from build123d import *

# Parameters (mm, degrees)
BOSS_EXTRUDE1_DEPTH = 1.6
SKETCH2_W           = 112.5
SKETCH2_H           = 91.209934792
BOSS_EXTRUDE2_DEPTH = 38
SKETCH3_W           = 129
SKETCH3_H           = 3
BOSS_EXTRUDE3_DEPTH = 38
SKETCH4_R           = 1.5
SKETCH4_R_2         = 1.75
CUT_EXTRUDE1_DEPTH  = 4
SKETCH5_R           = 1.75
SKETCH5_R_2         = 1.5
CUT_EXTRUDE2_DEPTH  = 4
FILLET1_R           = 2
FILLET2_R           = 2
FILLET3_R           = 2


with BuildPart() as part:
    # Sketch1 → Boss-Extrude1 (new body)
    with BuildSketch(Plane(origin=(0, 0, 0), x_dir=(1, 0, 0), z_dir=(0, 1, 0))):
        with BuildLine():
            Line((-68.019736842, 49), (-68.019736842, -49))
            Line((-68.019736842, -49), (60.980263158, -49))
            Line((60.980263158, -49), (60.980263158, -46))
            Line((60.980263158, -46), (54.480263158, -46))
            Line((54.480263158, -46), (54.480263158, 40.25))
            ThreePointArc((54.480263158, 40.25), (52.730263158, 42), (54.480263158, 43.75))
            Line((54.480263158, 43.75), (60.980263158, 43.75))
            Line((60.980263158, 43.75), (60.980263158, 49))
            Line((60.980263158, 49), (-68.019736842, 49))
        make_face()
    extrude(amount=BOSS_EXTRUDE1_DEPTH)

    # Sketch2 → Boss-Extrude2 (add)
    with BuildSketch(Plane(origin=(0, 1.6, 0), x_dir=(1, 0, 0), z_dir=(0, 1, 0))):
        with Locations((-5.269736842, -0.395032604)):
            Rectangle(SKETCH2_W, SKETCH2_H)
    extrude(amount=BOSS_EXTRUDE2_DEPTH)

    # Sketch3 → Boss-Extrude3 (add)
    with BuildSketch(Plane(origin=(0, 1.6, 0), x_dir=(1, 0, 0), z_dir=(0, 1, 0))):
        with Locations((-3.519736842, -47.5)):
            Rectangle(SKETCH3_W, SKETCH3_H)
    extrude(amount=BOSS_EXTRUDE3_DEPTH)

    # Sketch4 → Cut-Extrude1 (cut)
    with BuildSketch(Plane.XY.offset(49)):
        with Locations((-36.019736842, 21.1)):
            Circle(SKETCH4_R)
        with Locations((40.980263158, 12.1)):
            Circle(SKETCH4_R)
        with Locations((40.980263158, 30.1)):
            Circle(SKETCH4_R)
        with Locations((-61.519736842, 30.6)):
            Circle(SKETCH4_R_2)
    extrude(amount=-CUT_EXTRUDE1_DEPTH, mode=Mode.SUBTRACT)

    # Sketch5 → Cut-Extrude2 (cut)
    with BuildSketch(Plane.XZ):
        with Locations(Location((-63.519736842, 43.5, 0), (0, 0, 270))):
            Circle(SKETCH5_R)
        with Locations(Location((9.980263158, 18, 0), (0, 0, 270))):
            Circle(SKETCH5_R_2)
        with Locations(Location((9.980263158, -15, 0), (0, 0, 270))):
            Circle(SKETCH5_R_2)
    extrude(amount=-CUT_EXTRUDE2_DEPTH, mode=Mode.SUBTRACT)

    # Fillet1
    fillet1_edges = [part.edges().sort_by_distance(p)[0] for p in [
        (60.980263158, 0.8, -49),
    ]]
    fillet(fillet1_edges, radius=FILLET1_R)

    # Fillet2
    fillet2_edges = [part.edges().sort_by_distance(p)[0] for p in [
        (60.980263158, 39.6, 47.5),
    ]]
    fillet(fillet2_edges, radius=FILLET2_R)

    # Fillet3
    fillet3_edges = [part.edges().sort_by_distance(p)[0] for p in [
        (-68.019736842, 39.6, 47.5),
    ]]
    fillet(fillet3_edges, radius=FILLET3_R)


solid = part.part
Could you check a few things on this model? Use its own coordinates, in mm. A direction names the side the tool comes from. Give positions to 0.01 mm unless a question says otherwise; leave off trailing zeros. Order: outer loops, then holes, each group sorted by start corner. A loop starts at its lowest first (then second) coordinate and runs counter-clockwise, first axis right, second up.
1. Suppose I cut it at A-A (z = 43.5). List the corners of the cut face in (x, y) for me, plus the area to 3 significant figures.
2. I need wall thicknesses on L1, parallel to X at y = 2, z = -15; L2, parallel to Z at x = -52, y = 37; L3, parallel to X at y = 22, z = 21. Which ranges of each line are inside material? Lowest first, please.
3. Suppose I cut it at B-B (y = 21.1). List the corners of the cut face in (x, z) for me, plus the area to 3 significant figures.
4. Suppose I cut it at C-C (x = -18). List the corners of the cut face in (y, z) for me, plus the area to 3 significant figures.
5. Suppose I cut it at D-D (z = 18). List the corners of the cut face in (x, y) for me, plus the area to 3 significant figures.
6. We'd pull the mould along X, two halves only. Please class faces 1 (the cylindrical face through (10, 2, 19.5)), 2 (the flat face through (-68.02, 1, 22)), 3 (the flat face through (56, 20, 46)): pulls with the +X half, pulls with the -X half, needs draft (parallel to the pull), parting line crosses it, or undercut.
7. Will these pins go through, and if not, where does the flat tip stop? P1, Ø5, axis at x = -65, y = 30, coming from the -Z side; P2, Ø2.5, axis at x = 40.98, y = 30.1, coming from the +Z side; P3, Ø1, axis at x = -37.5, z = -15, coming from the -Y side; P4, Ø4, axis at y = 16.5, z = -33, coming from the -X side.
8. For faces 4 (the flat face through (41, 12, 45)), 5 (the flat face through (10, 4, -15)), 6 (the flat face through (-4, 1.6, -47)), 7 (the flat face through (-6, 20, -45.21)), which set-ups out of +Z, -Z, +X, -X, +Y, -Y let a thin tool reach every point of the face, with its end or its side?
Solved:
1. outline: (-68.02, 0) - (-65.27, 0) - (-65.27, 1.6) - (-68.02, 1.6) - close; (-61.77, 0) - (54.48, 0) - (54.48, 1.6) - (50.98, 1.6) - (50.98, 39.6) - (-61.52, 39.6) - (-61.52, 1.6) - (-61.77, 1.6) - close
1. area: 4,470 mm2
2. L1: x = -61.52 to 8.48, 11.48 to 50.98
2. L2: z = -45.21 to 49
2. L3: x = -61.52 to 50.98
3. outline: (-68.02, 46) - (-61.52, 46) - (-61.52, -45.21) - (50.98, -45.21) - (50.98, 46) - (60.98, 46) - (60.98, 49) - (-34.52, 49) - (-34.52, 45) - (-37.52, 45) - (-37.52, 49) - (-68.02, 49) - close
3. area: 10,600 mm2
4. outline: (0, -49) - (1.6, -49) - (1.6, -45.21) - (39.6, -45.21) - (39.6, 49) - (0, 49) - close
4. area: 3,740 mm2
5. outline: (-68.02, 0) - (8.48, 0) - (8.48, 4) - (11.48, 4) - (11.48, 0) - (54.48, 0) - (54.48, 1.6) - (50.98, 1.6) - (50.98, 39.6) - (-61.52, 39.6) - (-61.52, 1.6) - (-68.02, 1.6) - close
5. area: 4,460 mm2
6. face 1: undercut
6. face 2: pulls with the -X half
6. face 3: needs draft
7. P1: stops at z = 46
7. P2: stops at z = 45
7. P3: stops at y = 0
7. P4: stops at x = -61.52
8. face 4: +Z
8. face 5: -Y
8. face 6: -Z, +Y
8. face 7: -Z, +X, -X, +Y
